Geometry: final body of the model. Coordinates: model frame, mm. A direction names the side the tool comes from. Coordinates: 2 decimals unless noted, no trailing zeros. Order: outer loops, then holes, each group sorted by start corner. A loop starts at its lowest first (then second) coordinate and runs counter-clockwise, first axis right, second up. Notation, with made-up numbers: M 78,82.25 L 95,82.25 A28 cw 95,107.25 Z; hole C -32.75,82.25 d3. An arc over 180 degrees is marked long. Use CSV: the item, a comma, the result in double quotes. Start each with the question number.
1. Section query B-B on y = -1.25. Return the cut outline in (x, z) (3 decimals), and give its area (3 significant figures).
2. Section query A-A on x = 0. Return the cut outline in (y, z) (3 decimals).
3. Section query C-C on z = -20. Return the cut outline in (x, y).
4. Pull-direction query (X, two-part tool) for faces 5 (the cylindrical face through (-0.909, 5.435, -6.926)), 6 (the flat face through (7.915, -3.131, 13.71)), 7 (the flat face through (-15.29, -3.13, 16.16)); classes: pulls with the +X half, pulls with the -X half, needs draft (parallel to the pull), parting line crosses it, or undercut.
5. Set-up query: faces 1 (the flat face through (-6.35, -3, -21)), 2 (the cylindrical face through (-10.95, -3.13, 6.43)), 3 (the cylindrical face through (3.937, 5.175, -1.284)), 4 (the flat face through (0, -6.35, -5)). Return all of +Z, -Z, +X, -X, +Y, -Y with unobstructed straight access to the full face (end or side cutting, diameter ignored); none if empty.
6. Section query D-D on y = 9.25. Return the cut outline in (x, z) (1 decimal), and give its area (3 significant figures).
7. First-contact query: P1, Ø1.1, axis at x = -1, z = -0.5, coming from the -Y side; P2, Ø3, axis at x = -13.5, z = -7, coming from the +Y side; P3, Ø6, axis at y = 2.5, z = 20, coming from the +X side; P4, Ø4, axis at y = 3.5, z = -14.5, coming from the +X side. Flat tips, straight axial feed; report the tip coordinate or a pass-through.
8. Material intervals for line 1 (X direction, y = -0.25, z = 1.5); line 2 (X direction, y = -1.25, z = 4); line 3 (Z direction, x = 0, y = -5.2) (3 decimals), sorted ascending.
from build123d import *

# Parameters (mm, degrees)
SKETCH1_R           = 6.985
BOSS_EXTRUDE1_DEPTH = 10.9965998
CHAMFER5_SIZE       = 1
CHAMFER6_SIZE       = 0.500000016
SKETCH2_R           = 1.058078275
BOSS_EXTRUDE2_DEPTH = 6.35
FILLET1_R           = 1.000000032
SKETCH3_R           = 1.905
CUT_EXTRUDE1_DEPTH  = 2.54


with BuildPart() as part:
    # Sketch1 → Boss-Extrude1 (new body)
    with BuildSketch(Plane(origin=(0, 0, 0), x_dir=(1, 0, 0), z_dir=(0, 1, 0))):
        Circle(SKETCH1_R)
        with BuildLine():
            Line((-3.302, 1.905), (3.302, 1.905))
            ThreePointArc((3.302, 1.905), (3.937, 1.27), (3.302, 0.635))
            Line((3.302, 0.635), (2.67270889, 0.5588))
            ThreePointArc((2.67270889, 0.5588), (2.7305, 0), (2.67270889, -0.5588))
            Line((2.67270889, -0.5588), (3.374233059, -0.639121735))
            ThreePointArc((3.374233059, -0.639121735), (3.935968729, -1.30617528), (3.302, -1.905))
            Line((3.302, -1.905), (-3.302, -1.905))
            ThreePointArc((-3.302, -1.905), (-3.937, -1.27), (-3.302, -0.635))
            Line((-3.302, -0.635), (-2.67270889, -0.5588))
            ThreePointArc((-2.67270889, -0.5588), (-2.7305, 0), (-2.67270889, 0.5588))
            Line((-2.67270889, 0.5588), (-3.374233059, 0.639121735))
            ThreePointArc((-3.374233059, 0.639121735), (-3.935968729, 1.30617528), (-3.302, 1.905))
        make_face(mode=Mode.SUBTRACT)
    extrude(amount=BOSS_EXTRUDE1_DEPTH)

    # Chamfer5
    chamfer5_edges = [part.edges().sort_by_distance(p)[0] for p in [
        (-6.985, 10.9965998, 0),
    ]]
    chamfer(chamfer5_edges, length=CHAMFER5_SIZE)

    # Chamfer6
    chamfer6_edges = [part.edges().sort_by_distance(p)[0] for p in [
        (-2.7305, 10.9965998, 0),
        (-2.987354445, 10.9965998, 0.5969),
        (-3.937, 10.9965998, 1.27),
        (0, 10.9965998, 1.905),
        (3.935968729, 10.9965998, 1.30617528),
        (3.023470975, 10.9965998, 0.598960868),
        (2.7305, 10.9965998, 0),
        (2.987354445, 10.9965998, -0.5969),
        (3.937, 10.9965998, -1.27),
        (0, 10.9965998, -1.905),
        (-3.935968729, 10.9965998, -1.30617528),
        (-3.023470975, 10.9965998, -0.598960868),
    ]]
    chamfer(chamfer6_edges, length=CHAMFER6_SIZE)

    # Sketch2 → Boss-Extrude2 (add)
    with BuildSketch(Plane.XZ):
        with BuildLine():
            Line((-6.35, -24.593444248), (-6.35, -17.960512242))
            ThreePointArc((-6.35, -17.960512242), (-7.971122868, -17.302129933), (-9.525, -16.497783942))
            Line((-9.525, -16.497783942), (-6.35, -10.998522628))
            ThreePointArc((-6.35, -10.998522628), (0, -12.7), (6.35, -10.998522628))
            Line((6.35, -10.998522628), (9.525, -16.497783942))
            ThreePointArc((9.525, -16.497783942), (7.971122868, -17.302129933), (6.35, -17.960512242))
            Line((6.35, -17.960512242), (6.35, -24.593444248))
            ThreePointArc((6.35, -24.593444248), (21.997045256, -12.7), (24.473547486, 6.79746081))
            Line((24.473547486, 6.79746081), (18.729259867, 3.480994807))
            ThreePointArc((18.729259867, 3.480994807), (18.969645496, 1.747870067), (19.05, 0))
            Line((19.05, 0), (12.7, 0))
            ThreePointArc((12.7, 0), (10.998522628, 6.35), (6.35, 10.998522628))
            Line((6.35, 10.998522628), (9.525, 16.497783942))
            ThreePointArc((9.525, 16.497783942), (10.998522628, 15.554259867), (12.379259867, 14.479517435))
            Line((12.379259867, 14.479517435), (18.123547486, 17.795983438))
            ThreePointArc((18.123547486, 17.795983438), (0, 25.4), (-18.123547486, 17.795983438))
            Line((-18.123547486, 17.795983438), (-12.379259867, 14.479517435))
            ThreePointArc((-12.379259867, 14.479517435), (-10.998522628, 15.554259867), (-9.525, 16.497783942))
            Line((-9.525, 16.497783942), (-6.35, 10.998522628))
            ThreePointArc((-6.35, 10.998522628), (-10.998522628, 6.35), (-12.7, 0))
            Line((-12.7, 0), (-19.05, 0))
            ThreePointArc((-19.05, 0), (-18.969645496, 1.747870067), (-18.729259867, 3.480994807))
            Line((-18.729259867, 3.480994807), (-24.473547486, 6.79746081))
            ThreePointArc((-24.473547486, 6.79746081), (-21.997045256, -12.7), (-6.35, -24.593444248))
        make_face()
        Circle(SKETCH2_R, mode=Mode.SUBTRACT)
    extrude(amount=BOSS_EXTRUDE2_DEPTH)

    # Fillet1
    fillet1_edges = [part.edges().sort_by_distance(p)[0] for p in [
        (-6.985, 0, 0),
    ]]
    fillet(fillet1_edges, radius=FILLET1_R)

    # Sketch3 → Cut-Extrude1 (cut)
    with BuildSketch(Plane.XZ.offset(6.35)):
        Circle(SKETCH3_R)
    extrude(amount=-CUT_EXTRUDE1_DEPTH, mode=Mode.SUBTRACT)


solid = part.part
Results list:
1,outline,"M -24.474,6.797 A25.4 ccw -6.35,-24.593 L -6.35,-17.961 A19.05 cw -9.525,-16.498 L -6.35,-10.999 A12.7 ccw 6.35,-10.999 L 9.525,-16.498 A19.05 cw 6.35,-17.961 L 6.35,-24.593 A25.4 ccw 24.474,6.797 L 18.729,3.481 A19.05 cw 19.05,0 L 12.7,0 A12.7 ccw 6.35,10.999 L 9.525,16.498 A19.05 cw 12.379,14.48 L 18.124,17.796 A25.4 ccw -18.124,17.796 L -12.379,14.48 A19.05 cw -9.525,16.498 L -6.35,10.999 A12.7 ccw -12.7,0 L -19.05,0 A19.05 cw -18.729,3.481 Z; hole C 0,0 d2.116"
1,area,"1,460 mm²"
2,outline,"M -6.35,-12.7 L 0,-12.7 L 0,-7.985 A1 cw 1,-6.985 L 9.997,-6.985 L 10.997,-5.985 L 10.997,-2.405 L 10.497,-1.905 L 0,-1.905 L 0,-1.058 L -3.81,-1.058 L -3.81,-1.905 L -6.35,-1.905 Z; M -6.35,1.905 L -3.81,1.905 L -3.81,1.058 L 0,1.058 L 0,1.905 L 10.497,1.905 L 10.997,2.405 L 10.997,5.985 L 9.997,6.985 L 1,6.985 A1 cw 0,7.985 L 0,25.4 L -6.35,25.4 Z"
3,outline,"M -15.66,-6.35 L -6.35,-6.35 L -6.35,0 L -15.66,0 Z; M 6.35,-6.35 L 15.66,-6.35 L 15.66,0 L 6.35,0 Z"
4,face 5,"parting line crosses it"
4,face 6,"undercut"
4,face 7,"pulls with the -X half"
5,face 1,"-Z, +Y, -Y"
5,face 2,"+Y, -Y"
5,face 3,"+Y"
5,face 4,"+Z, -Z, +X, -X, -Y"
6,outline,"C 0,0 d14; hole M -3.4,-0.6 A0.6 ccw -3.3,-1.9 L 3.3,-1.9 A0.6 ccw 3.3,-0.6 L 2.7,-0.6 A2.7 ccw 2.7,0.6 L 3.4,0.6 A0.6 ccw 3.3,1.9 L -3.3,1.9 A0.6 ccw -3.3,0.6 L -2.7,0.6 A2.7 ccw -2.7,-0.6 Z"
6,area,"127 mm²"
7,P1,"stops at y = -3.81"
7,P2,"stops at y = 0"
7,P3,"stops at x = 17.57"
7,P4,"passes through"
8,line 1,"x = -25.36 to -18.99, -12.61 to 12.61, 18.99 to 25.36"
8,line 2,"x = -25.08 to -19.63, -12.05 to 12.05, 19.63 to 25.08"
8,line 3,"z = -12.7 to -1.905, 1.905 to 25.4"
